Check sheet for the modelled part. Datum: model origin and axes. Units: mm. Round coordinates to 2 decimals unless told otherwise and drop trailing zeros. Write each loop counter-clockwise with the first axis right and the second up, starting at its lowest first coordinate (ties: lowest second). Pieces come first, ordered by that corner, then holes. Notation, with made-up numbers: (-16.75, 8) -> (30.25, 8) arc R13 cw to (30.25, 25) -> close; hole circle Ø5 at (5, -27.5). An arc over 180 degrees is marked (long way). Answer as a JSON object with one key per item and string values. Group by question number.
Autodesk Inventor part; units mm, degrees
ref_plane "YZ Plane" through (0, 0, 0) normal (1, 0, 0) x (0, 1, 0)
ref_plane "XZ Plane" through (0, 0, 0) normal (0, 1, 0) x (-1, 0, 0)
ref_plane "XY Plane" through (0, 0, 0) normal (0, 0, 1) x (1, 0, 0)
sketch "Sketch1" plane through (0, 0, 0) normal (0, 1, 0) x (-1, 0, 0)
  line L0 (13.2677, 19.6408) -> (-12.1323, 19.6408)
  line L1 (-12.1323, 19.6408) -> (-12.1323, -18.4592)
  line L2 (-12.1323, -18.4592) -> (13.2677, -18.4592)
  line L3 (13.2677, -18.4592) -> (13.2677, 19.6408)
  point P0 (0, 0)
  dimension "d0" = 25.4
  dimension "d1" = 38.1
extrude "Extrusion1" add sketch "Sketch1" along normal blind 3.175
hole "Hole1" at (-9.6799, 3.175, 14.8783) direction (0, -1, 0) diameter 4.4958 depth 3.175
hole "Hole2" at (8.5446, 3.175, 14.8783) direction (0, -1, 0) diameter 4.4958 depth 3.175
hole "Hole3" at (-9.6799, 3.175, -13.6967) direction (0, -1, 0) diameter 4.4958 depth 3.175
hole "Hole4" at (8.5446, 3.175, -13.6967) direction (0, -1, 0) diameter 4.4958 depth 3.175
sketch "Sketch2" plane through (0, 3.175, 0) normal (0, 1, 0) x (1, 0, 0)
  circle A0 centre (0, 0) radius 3.175
  dimension "d58" = 6.35
extrude "Extrusion2" add sketch "Sketch2" along normal blind 304.8
sketch "Sketch3" plane through (0, 0, 0) normal (1, 0, 0) x (0, 1, 0)
  point P0 (0, 0)
sketch "Sketch4" plane through (0, 307.975, 0) normal (0, 1, 0) x (1, 0, 0)
  circle A0 centre (0, 0) radius 3.175
extrude "Extrusion3" add sketch "Sketch4" along normal blind 63.5
sketch "Sketch5" plane through (0, 0, 0) normal (1, 0, 0) x (0, 1, 0)
  point P0 (0, 0)
sketch "Sketch6" plane through (0, 371.475, 0) normal (0, 1, 0) x (1, 0, 0)
  circle A0 centre (0, 0) radius 3.175
extrude "Extrusion4" cut sketch "Sketch6" against normal blind 139.7
properties part number "rotatable rod table"
(1) Scan lines: line 1 along Y through (x, z) = (-7, 15) (3 decimals); line 2 along X through (y, z) = (170.5, 0.5); line 3 along Z through (x, y) = (1.5, 218). Record each from-to range of solid material in increasing order.
(2) Section check C-C on y = 33. Record the cut outline in (x, z) (3 decimals), then the cut area to 3 significant figures.
(3) Release check for a two-part mould opening along Z. For faces 1 (the cylindrical face through (-0.69, 115.87, -3.1)), 2 (the cylindrical face through (8.446, 1.565, 12.633)), 3 (the flat face through (0, 0, 1)) record: pulls with the +Z half, pulls with the -Z half, needs draft (parallel to the pull), parting line crosses it, or undercut.
(4) Section check A-A on z = 0. Record the cut outline in (x, y) (3 decimals), then the cut area to 3 significant figures.
(5) Go/stop test with flat-tipped pins: pin 1 Ø7 at (x, z) = (-9.68, 14.88) entering from +Y (3 decimals); pin 2 Ø4 at (x, z) = (8.54, 14.88) entering from +Y; pin 3 Ø3 at (x, y) = (3, 189.5) entering from -Z; pin 4 Ø12 at (x, y) = (-6, 53.5) entering from -Z (3 decimals). Record where each tip stops, or that it passes through.
(6) Section check B-B on x = 0. Record the cut outline in (y, z) (3 decimals).
Data:
{
 "1": {"line 1": "y = 0 to 3.175", "line 2": "x = -3.14 to 3.14", "line 3": "z = -2.8 to 2.8"},
 "2": {"outline": "circle Ø6.35 at (0, 0)", "area": "31.7 mm²"},
 "3": {"face 1": "parting line crosses it", "face 2": "undercut", "face 3": "needs draft"},
 "4": {"outline": "(-13.268, 0) -> (12.132, 0) -> (12.132, 3.175) -> (3.175, 3.175) -> (3.175, 231.775) -> (-3.175, 231.775) -> (-3.175, 3.175) -> (-13.268, 3.175) -> close", "area": "1,530 mm²"},
 "5": {"pin 1": "stops at y = 3.175", "pin 2": "passes through", "pin 3": "stops at z = -2.8", "pin 4": "stops at z = -3.175"},
 "6": {"outline": "(0, -18.459) -> (3.175, -18.459) -> (3.175, -3.175) -> (231.775, -3.175) -> (231.775, 3.175) -> (3.175, 3.175) -> (3.175, 19.641) -> (0, 19.641) -> close"}
}
